Can you work these out from the drawing? Everything is in mm from the part's minimum corner. A direction names the side the tool comes from. Give positions to 0.01 mm unless a question says otherwise; leave off trailing zeros. Loops run counter-clockwise (first coordinate to the right, second up) from the corner with the lowest first, then second, coordinate; pieces in that order, holes last.
Q1. Will these pins go through, and if not, where does the flat tip stop? P1, Ø10, axis at x = 2.5, y = 2.5, coming from the -Z side; P2, Ø5, axis at y = 18.5, z = 4.5, coming from the -X side; P3, Ø1, axis at y = 14, z = 8, coming from the -X side; P4, Ø2, axis at x = 11, y = 19, coming from the -Z side.
Q2. If we section it at A-A (x = 11): Please give me the cut outline in (y, z).
Q3. We'd pull the mould along Y, two halves only. Please class the marked faces 4, 5, 6 and 7: +Y half, -Y half, draft (parallel to the pull), parting line (faces both ways), or undercut.
Q4. If we section it at C-C (y = 18.5): Please give me the cut outline in (x, z), plus the area to 3 significant figures.
Q5. For the marked faces 1, 2 and 3, which set-ups out of +Z, -Z, +X, -X, +Y, -Y let a thin tool reach every point of the face, with its end or its side?
Q6. If we section it at D-D (z = 12.75): Please give me the cut outline in (x, y), plus the area to 3 significant figures.
Q7. I need wall thicknesses on line 1 (Y direction, x = 11, z = 12.95); line 2 (Z direction, x = 4.5, y = 14.75); line 3 (X direction, y = 3, z = 12.95). Which ranges of each line are inside material? Lowest first, please.
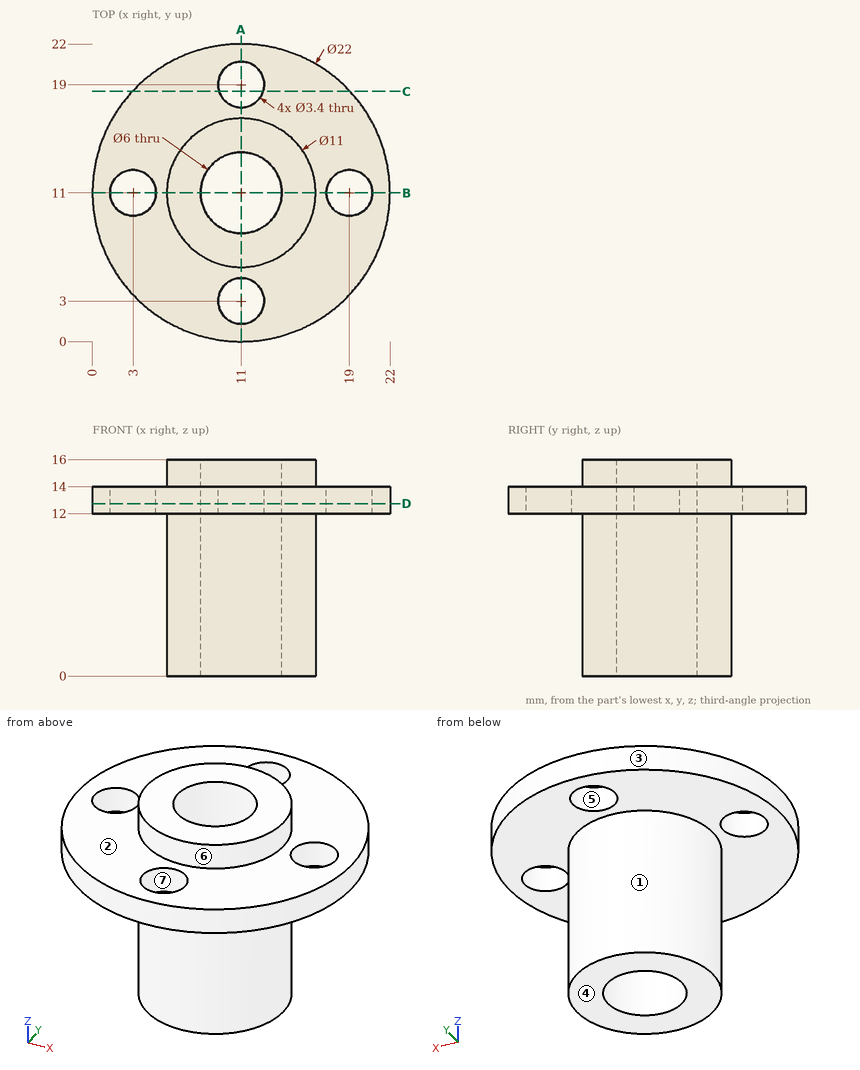
Check sheet entries:
1. P1: stops at z = 12
1. P2: stops at x = 8.71
1. P3: stops at x = 6.1
1. P4: passes through
2. outline: (0, 12) - (1.3, 12) - (1.3, 14) - (0, 14) - close; (4.7, 12) - (5.5, 12) - (5.5, 0) - (8, 0) - (8, 16) - (5.5, 16) - (5.5, 14) - (4.7, 14) - close; (14, 0) - (16.5, 0) - (16.5, 12) - (17.3, 12) - (17.3, 14) - (16.5, 14) - (16.5, 16) - (14, 16) - close; (20.7, 12) - (22, 12) - (22, 14) - (20.7, 14) - close
3. face 4: draft
3. face 5: undercut
3. face 6: parting line
3. face 7: undercut
4. outline: (2.95, 12) - (9.38, 12) - (9.38, 14) - (2.95, 14) - close; (12.62, 12) - (19.05, 12) - (19.05, 14) - (12.62, 14) - close
4. area: 25.7 mm2
5. face 1: -Z
5. face 2: +Z
5. face 3: +Z, -Z
6. outline: circle Ø22 at (11, 11); hole circle Ø3.4 at (3, 11); hole circle Ø6 at (11, 11); hole circle Ø3.4 at (11, 3); hole circle Ø3.4 at (11, 19); hole circle Ø3.4 at (19, 11)
6. area: 316 mm2
7. line 1: y = 0 to 1.3, 4.7 to 8, 14 to 17.3, 20.7 to 22
7. line 2: z = 12 to 14
7. line 3: x = 3.45 to 9.3, 12.7 to 18.55
